Autodesk Inventor part; units mm, degrees
ref_plane "YZ Plane" through (0, 0, 0) normal (1, 0, 0) x (0, 1, 0)
ref_plane "XZ Plane" through (0, 0, 0) normal (0, 1, 0) x (-1, 0, 0)
ref_plane "XY Plane" through (0, 0, 0) normal (0, 0, 1) x (1, 0, 0)
sketch "Sketch1" plane through (0, 0, 0) normal (0, 0, 1) x (1, 0, 0)
  line L0 (0, 0) -> (161.3408, 0)
  line L1 (161.3408, 0) -> (161.3408, 107.95)
  line L2 (161.3408, 107.95) -> (0, 107.95)
  line L3 (0, 107.95) -> (0, 0)
  line L4 (3.175, 3.175) -> (158.1658, 3.175)
  line L5 (158.1658, 3.175) -> (158.1658, 104.775)
  line L6 (158.1658, 104.775) -> (3.175, 104.775)
  line L7 (3.175, 104.775) -> (3.175, 3.175)
  dimension "d0" = 161.3408
  dimension "d1" = 107.95
  dimension "d2" = 154.9908
  dimension "d3" = 101.6
  dimension "d4" = 3.175
  dimension "d5" = 3.175
extrude "Extrusion1" add sketch "Sketch1" against normal blind 180.34
sketch "Sketch2" plane through (161.3408, 0, 0) normal (1, 0, 0) x (0, 0, -1)
  line L0 (0, 3.175) -> (180.34, 3.175)
  line L1 (0, 107.95) -> (180.34, 107.95)
  line L2 (0, 3.175) -> (76.2, 3.175)
  line L3 (76.2, 3.175) -> (76.2, 107.95)
  line L4 (76.2, 107.95) -> (0, 107.95)
  line L5 (0, 107.95) -> (0, 3.175)
  point P0 (0, 0)
  dimension "d8" = 76.2
extrude "Extrusion2" cut sketch "Sketch2" against normal through all
properties part number "Bucket" material "Polycarbonate, Clear"
CAD build for the part. Positions are in the model's coordinates, mm. A direction names the side the tool comes from. Round coordinates to 2 decimals unless told otherwise and drop trailing zeros. Write each loop counter-clockwise with the first axis right and the second up, starting at its lowest first coordinate (ties: lowest second). Pieces come first, ordered by that corner, then holes. Notation, with made-up numbers: M -38,7 L -30,7 A22 ccw -30,33 Z; hole C -6,-17 d6. An arc over 180 degrees is marked long. Put each result on its own line as item: value. Start each with the question number.
1) Drill centre lines: probe 1 along Y at (x, z) = (145, -151) (3 decimals); probe 2 along X at (y, z) = (95, -129.5) (3 decimals); probe 3 along Y at (x, z) = (112, -72) (3 decimals). Where is each one in solid material? Low to high. Write a range as [from, to].
2) 3-axis set-ups, long thin cutter, end or side, ignore diameter. For faces 4 (the flat face through (117, 106, -76.2)), 5 (the flat face through (3.175, 55, -128)), 6 (the flat face through (80, 0, -89)): which of +Z, -Z, +X, -X, +Y, -Y reach the whole face in a straight line?
3) Pull direction X, two halves, no side cores. Call faces 1 (the flat face through (161.341, 53, -129)), 2 (the flat face through (158.166, 53, -128)), 3 (the flat face through (82, 107.95, -128)): pulls with the +X half, pulls with the -X half, needs draft (parallel to the pull), parting line crosses it, or undercut.
4) Saw through at C-C, the plane z = -110. Write the cut outline in (x, y) (3 decimals), and give its area (3 significant figures).
5) Pin check, flat tips, straight feed: pin 1 Ø4 at (x, z) = (53, -79.5) entering from -Y; pin 2 Ø1 at (x, z) = (87.5, -72) entering from +Y (3 decimals). Stop position of each tip, or through.
6) Saw through at B-B, the plane x = 101.5. Write the cut outline in (y, z) (3 decimals).
7) Saw through at D-D, the plane z = -58.5. Write the cut outline in (x, y) (3 decimals).
8) Saw through at A-A, the plane y = 64.5. Write the cut outline in (x, z) (3 decimals), and give its area (3 significant figures).
Resolved:
1. probe 1: [0, 3.175], [104.775, 107.95]
1. probe 2: [0, 3.175], [158.166, 161.341]
1. probe 3: [0, 3.175]
2. face 4: +Z, +X, -X, +Y
2. face 5: +Z, -Z
2. face 6: +Z, -Z, +X, -X, -Y
3. face 1: pulls with the +X half
3. face 2: undercut
3. face 3: needs draft
4. outline: M 0,0 L 161.341,0 L 161.341,107.95 L 0,107.95 Z; hole M 3.175,3.175 L 158.166,3.175 L 158.166,104.775 L 3.175,104.775 Z
4. area: 1,670 mm²
5. pin 1: y = 0
5. pin 2: y = 3.175
6. outline: M 0,-180.34 L 3.175,-180.34 L 3.175,0 L 0,0 Z; M 104.775,-180.34 L 107.95,-180.34 L 107.95,-76.2 L 104.775,-76.2 Z
7. outline: M 0,0 L 161.341,0 L 161.341,3.175 L 0,3.175 Z
8. outline: M 0,-180.34 L 3.175,-180.34 L 3.175,-76.2 L 0,-76.2 Z; M 158.166,-180.34 L 161.341,-180.34 L 161.341,-76.2 L 158.166,-76.2 Z
8. area: 661 mm²
